Check sheet for the modelled part. Datum: model origin and axes. Units: mm. Give positions to 0.01 mm unless a question says otherwise; leave off trailing zeros. Order: outer loops, then holes, each group sorted by start corner. A loop starts at its lowest first (then second) coordinate and runs counter-clockwise, first axis right, second up. Notation, with made-up numbers: M 9,-2.75 L 19,-2.75 A25 cw 19,11.25 Z; hole C -3,14 d3. An arc over 180 degrees is marked long. Return JSON: item names as keys, results as strings. Group by question number.
from build123d import *

# Parameters (mm, degrees)
BOSS_EXTRUDE1_DEPTH     = 3.175
F_1_4_CLEARANCE_HOLE1_D = 6.7564
SKETCH7_W               = 1828.8
SKETCH7_H               = 50.8
BOSS_EXTRUDE3_DEPTH     = 3.175


with BuildPart() as part:
    # Sketch1 → Boss-Extrude1 (new body)
    with BuildSketch(Plane.XY):
        Polygon((0, 0), (1828.8, 1117.6), (1828.8, 0), align=None)
    extrude(amount=BOSS_EXTRUDE1_DEPTH)

    # 1/4 Clearance Hole1 (through all)
    with Locations(Plane(origin=(0, 0, 0), x_dir=(-1, 0, 0), z_dir=(0, 0, -1))):
        with Locations((-1816.1, 77.7875), (-1816.1, 399.520833333), (-1816.1, 721.254166667), (-1816.1, 1042.9875), (-1701.8, 19.05), (-1701.8, 57.15), (-1257.3, 57.15), (-1257.3, 19.05), (-533.4, 57.15), (-533.4, 19.05), (-127, 57.15), (-127, 19.05)):
            Hole(F_1_4_CLEARANCE_HOLE1_D / 2)

    # Sketch7 → Boss-Extrude3 (add)
    with BuildSketch(Plane(origin=(0, 0, 0), x_dir=(-1, 0, 0), z_dir=(0, 0, -1))):
        with Locations((-914.4, -25.4)):
            Rectangle(SKETCH7_W, SKETCH7_H)
    extrude(amount=-BOSS_EXTRUDE3_DEPTH)


solid = part.part
1) Sectioned sample at A-A on z = 1.6. State how many separate pieces and enclosed holes the cut face has, then the cut area to 3 significant figures.
2) Depth check by flat-ended pin: P1, Ø8, axis at x = 1816.1, y = 721.25, coming from the +Z side (3 decimals); P2, Ø1, axis at y = 531.5, z = 0.5, coming from the -X side; P3, Ø1, axis at y = 126, z = 2.5, coming from the -X side. Enter the tip coordinate at first touch or a pass-through.
3) Sectioned sample at C-C on x = 740. Record the boundary of the cut face in (y, z) (3 decimals).
4) Sectioned sample at B-B on y = 297. Record the boundary of the cut face in (x, z) (3 decimals), then the cut area to 3 significant figures.
5) Material ranges on line 1 along Y through (x, z) = (127, 1.65); line 2 along Y through (x, z) = (125.5, 1.05); line 3 along Y through (x, z) = (1816.1, 1.4), recorded low to high.
Reply:
{
 "1": {"separate pieces": "1", "enclosed holes": "12", "area": "1,110,000 mm^2"},
 "2": {"P1": "z = 3.175", "P2": "x = 868.91", "P3": "x = 205.36"},
 "3": {"outline": "M -50.8,0 L 452.222,0 L 452.222,3.175 L -50.8,3.175 Z"},
 "4": {"outline": "M 486,0 L 1828.8,0 L 1828.8,3.175 L 486,3.175 Z", "area": "4,260 mm^2"},
 "5": {"line 1": "-50.8 to 15.67, 22.43 to 53.77, 60.53 to 77.61", "line 2": "-50.8 to 16.02, 22.08 to 54.12, 60.18 to 76.69", "line 3": "-50.8 to 74.41, 81.17 to 396.14, 402.9 to 717.88, 724.63 to 1039.61, 1046.37 to 1109.84"}
}
